Check sheet for the modelled part. Datum: model origin and axes. Units: mm. Face numbers are marked on the shaded views. A direction names the side the tool comes from. Give positions to 0.01 mm unless a question says otherwise; leave off trailing zeros. Order: outer loops, then holes, each group sorted by start corner. A loop starts at its lowest first (then second) coordinate and runs counter-clockwise, first axis right, second up.
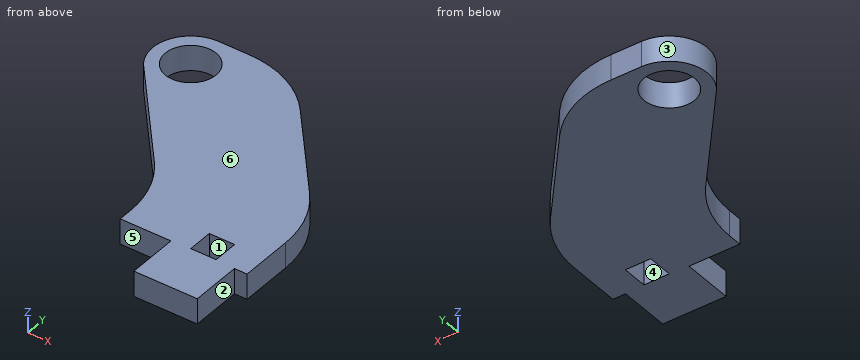
```python
from build123d import *

# Parameters (mm, degrees)
SKETCH1_R           = 3.175
BOSS_EXTRUDE1_DEPTH = 3.175
CUT_EXTRUDE1_REACH  = 5.175
SKETCH2_W           = 3.175
SKETCH2_H           = 3.175
FILLET1_R           = 12.7


with BuildPart() as part:
    # Sketch1 → Boss-Extrude1 (new body)
    with BuildSketch(Plane.XY):
        with BuildLine():
            Line((-3.96875, 0), (3.96875, 0))
            Line((3.96875, 0), (3.96875, 6.35))
            Line((3.96875, 6.35), (5.55625, 6.35))
            Line((5.55625, 6.35), (5.55625, 17.564325962))
            Line((5.55625, 17.564325962), (-10.31875, 36.5125))
            Line((-10.31875, 36.5125), (-20.066, 36.5125))
            ThreePointArc((-20.066, 36.5125), (-24.38152939, 33.764351592), (-23.716600944, 28.691484184))
            Line((-23.716600944, 28.691484184), (-10.31875, 12.7))
            Line((-10.31875, 12.7), (-10.31875, 6.35))
            Line((-10.31875, 6.35), (-3.96875, 6.35))
            Line((-3.96875, 6.35), (-3.96875, 0))
        make_face()
        with Locations((-20.066, 31.75)):
            Circle(SKETCH1_R, mode=Mode.SUBTRACT)
    extrude(amount=BOSS_EXTRUDE1_DEPTH)

    # Sketch2 → Cut-Extrude1 (cut, up to next)
    with BuildSketch(Plane.XY.offset(3.175), mode=Mode.PRIVATE) as cut_extrude1_sk1:
        with Locations((0, 8.0645)):
            Rectangle(SKETCH2_W, SKETCH2_H)
    cut_extrude1_tool1 = extrude(cut_extrude1_sk1.sketch, amount=-CUT_EXTRUDE1_REACH, mode=Mode.PRIVATE) & part.part
    add(cut_extrude1_tool1.solids().sort_by_distance((0, 8.0645, 3.175))[0], mode=Mode.SUBTRACT)

    # Fillet1
    fillet1_edges = [part.edges().sort_by_distance(p)[0] for p in [
        (-10.31875, 12.7, 1.5875),
        (-10.31875, 36.5125, 1.5875),
        (5.55625, 17.564325962, 1.5875),
    ]]
    fillet(fillet1_edges, radius=FILLET1_R)


solid = part.part
```
(1) Release check for a two-part mould opening along X. For the marked faces 1, 2 and 3 record: released by +X, released by -X, zero draft, split by the parting line, or undercut.
Response values:
face 1: undercut
face 2: released by +X
face 3: released by -X
(2) Gauge pin test, flat ends, axial feed: pin 1 Ø12 at (x, y) = (-18, 10) entering from +Z; pin 2 Ø1.6 at (x, z) = (0, 2) entering from +Y; pin 3 Ø0.8 at (x, z) = (4.5, 1.5) entering from -Y; pin 4 Ø1.6 at (y, z) = (9, 1.5) entering from -X. Record the tip position at first contact, or that the pin passes through.
Response values:
pin 1: passes through
pin 2: stops at y = 25.15
pin 3: stops at y = 6.35
pin 4: stops at x = -10.44
(3) Set-up check for the marked faces 4, 5 and 6: record each of +Z, -Z, +X, -X, +Y, -Y from which the full face is reachable in a straight line by a thin tool's end or side.
Response values:
face 4: +Z, -Z
face 5: +Z, -Z, -X, -Y
face 6: +Z, +X, -X, +Y, -Y
(4) Cross-section at A-A on z = 2. Count the separate pieces of the cut face and the enclosed holes in it, then the cut area to 3 significant figures.
Response values:
separate pieces: 1
enclosed holes: 2
area: 547 mm2
(5) Cross-section at B-B on y = 18. Enter the section's corners in (x, z) (3 decimals).
Response values:
outline: (-14.759, 0) - (4.508, 0) - (4.508, 3.175) - (-14.759, 3.175) - close
(6) Cross-section at C-C on x = -6. Enter the section's corners in (y, z) (3 decimals).
Response values:
outline: (6.35, 0) - (31.358, 0) - (31.358, 3.175) - (6.35, 3.175) - close
(7) Material ranges on L1, parallel to X at y = 9, z = 1.7; L2, parallel to X at y = 3.5, z = 0.95; L3, parallel to X at y = 32.5, z = 1.9, recorded low to high.
Response values:
L1: x = -10.35 to -1.59, 1.59 to 5.56
L2: x = -3.97 to 3.97
L3: x = -24.77 to -23.15, -16.98 to -6.98
